Input: part model. Units: mm. Frame: model coordinates. Face numbers are marked on the shaded views. A direction names the side the tool comes from. Give positions to 0.01 mm unless a question says otherwise; leave off trailing zeros. Loops run counter-clockwise (first coordinate to the right, second up) from the corner with the lowest first, then second, coordinate; pieces in that order, holes last. Notation, with made-up numbers: (31, -7) -> (59, -7) arc R12 ccw to (59, 13) -> close; hole circle Ø3 at (89.5, 8). An arc over 180 degrees is marked (long way). Use CSV: the item, a comma, the result in double quotes.
```python
from build123d import *

# Parameters (mm, degrees)
F1_DEPTH = 228.6
F3_DEPTH = 228.6


with BuildPart() as f1:
    # F0 (on Front) → F1 (new body)
    with BuildSketch(Plane.XZ):
        Polygon((-63.258275, -30.340541), (-30.223398, -16.986018), (-63.258275, 0), align=None)
    extrude(amount=F1_DEPTH)

    # F2 (on Front) → F3 (join)
    with BuildSketch(Plane.XZ):
        Polygon((-7.028698, 0), (-30.691978, -17.220307), (-7.028698, -29.403383), align=None)
    extrude(amount=F3_DEPTH)


solid = f1.part
```
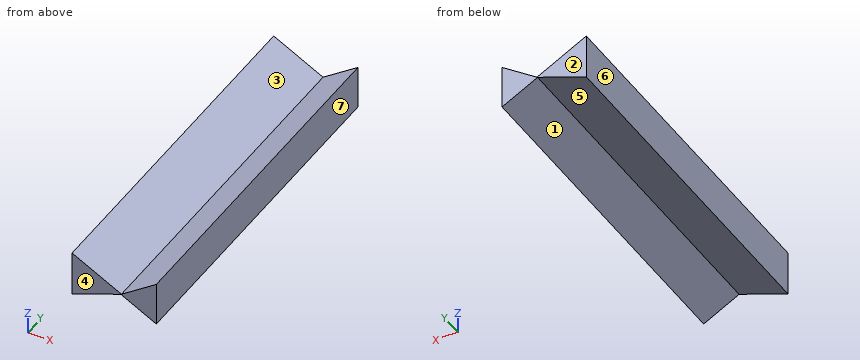
1) Mould query, pull axis X, two halves, no side actions, for the marked faces 4, 5, 6 and 7. Classes: pulls with the +X half, pulls with the -X half, needs draft (parallel to the pull), parting line crosses it, or undercut.
From the geometry:
face 4,"needs draft"
face 5,"undercut"
face 6,"pulls with the -X half"
face 7,"pulls with the +X half"
2) Section query C-C (z = -5). Return loops of the section in (x, y).
From the geometry:
outline,"(-63.26, -228.6) -> (-53.53, -228.6) -> (-53.53, 0) -> (-63.26, 0) -> close; (-13.9, -228.6) -> (-7.03, -228.6) -> (-7.03, 0) -> (-13.9, 0) -> close"
3) Ray query, line 1 (X direction, y = -193, z = -23); line 2 (X direction, y = -19, z = -29); line 3 (Z direction, x = -40, y = -203). Return the intervals inside material, ascending.
From the geometry:
line 1,"x = -63.26 to -45.1, -19.47 to -7.03"
line 2,"x = -63.26 to -59.94, -7.81 to -7.03"
line 3,"z = -20.94 to -11.96"
4) Contact query for flat-ended pins moving along their axis: pin 1 (10 mm diameter, centred on x = -26.5, y = -200, fed in from +Z); pin 2 (5 mm diameter, centred on x = -53.5, y = -91.5, fed in from +Z); pin 3 (4 mm diameter, centred on x = -39, z = -8.5, fed in from +Y) (3 decimals); pin 4 (1 mm diameter, centred on x = -13.5, y = -110.5, fed in from +Z). Output: stop coordinate, or through.
From the geometry:
pin 1,"stops at z = -10.53"
pin 2,"stops at z = -3.73"
pin 3,"passes through"
pin 4,"stops at z = -4.35"
5) Section query B-B (y = -56.5). Return loops of the section in (x, z).
From the geometry:
outline,"(-63.26, -30.34) -> (-30.55, -17.12) -> (-30.69, -17.22) -> (-7.03, -29.4) -> (-7.03, 0) -> (-30.31, -16.94) -> (-63.26, 0) -> close"
6) Reachability of the marked faces 1, 2 and 3 from +Z, -Z, +X, -X, +Y, -Y: full face, straight path, thin tool, end or side. Return the list, or none.
From the geometry:
face 1,"-Z, +Y, -Y"
face 2,"+Z, -Z, +X, -X, +Y"
face 3,"+Z, +Y, -Y"
7) Section query D-D (x = -35.5). Return loops of the section in (y, z).
From the geometry:
outline,"(-228.6, -19.12) -> (0, -19.12) -> (0, -14.27) -> (-228.6, -14.27) -> close"
8) Section query A-A (z = -15). Return loops of the section in (x, y).
From the geometry:
outline,"(-63.26, -228.6) -> (-34.09, -228.6) -> (-34.09, 0) -> (-63.26, 0) -> close; (-27.64, -228.6) -> (-7.03, -228.6) -> (-7.03, 0) -> (-27.64, 0) -> close"
